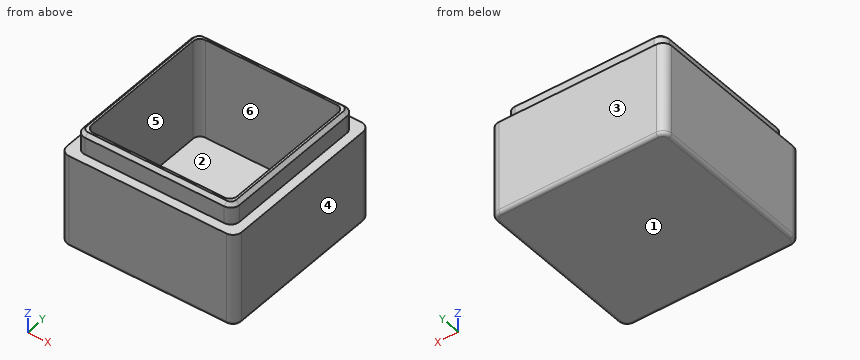
from build123d import *

# Parameters (mm, degrees)
F0_W          = 50.5
F0_H          = 50.5
F1_DEPTH      = 27
F2_W          = 45.2
F2_H          = 45.2
F3_DEPTH      = 6
F4_W          = 42
F4_H          = 42
F5_DEPTH      = 6
F5_DEPTH_BACK = 23
F6_R          = 2.5
F7_R          = 2
F8_SIZE       = 1
F9_R          = 1


with BuildPart() as f1:
    # F0 (on Top) → F1 (new body)
    with BuildSketch(Plane.XY):
        Rectangle(F0_W, F0_H)
    extrude(amount=F1_DEPTH)

    # F2 (on face) → F3 (join)
    with BuildSketch(Plane.XY.offset(27)):
        Rectangle(F2_W, F2_H)
    extrude(amount=F3_DEPTH)

    # F4 (on face) → F5 (cut, two sides)
    with BuildSketch(Plane.XY.offset(27)) as f5_sk:
        Rectangle(F4_W, F4_H)
    extrude(amount=F5_DEPTH, mode=Mode.SUBTRACT)
    extrude(f5_sk.sketch, amount=-F5_DEPTH_BACK, mode=Mode.SUBTRACT)

    # F6
    f6_edges = [f1.edges().sort_by_distance(p)[0] for p in [
        (-25.25, 25.25, 13.5),
        (-25.25, -25.25, 13.5),
        (25.25, -25.25, 13.5),
        (25.25, 25.25, 13.5),
        (-22.6, 22.6, 30),
        (-22.6, -22.6, 30),
        (22.6, -22.6, 30),
        (22.6, 22.6, 30),
    ]]
    fillet(f6_edges, radius=F6_R)

    # F7
    f7_edges = [f1.edges().sort_by_distance(p)[0] for p in [
        (-21, 21, 18.5),
        (21, 21, 18.5),
        (21, -21, 18.5),
        (-21, -21, 18.5),
    ]]
    fillet(f7_edges, radius=F7_R)

    # F8
    f8_edges = [f1.edges().sort_by_distance(p)[0] for p in [
        (-22.6, 0, 33),
    ]]
    chamfer(f8_edges, length=F8_SIZE)

    # F9
    f9_edges = [f1.edges().sort_by_distance(p)[0] for p in [
        (0, 25.25, 0),
    ]]
    fillet(f9_edges, radius=F9_R)


solid = f1.part
Check sheet for the modelled part. Datum: model origin and axes. Units: mm. Face numbers are marked on the shaded views. A direction names the side the tool comes from. Give positions to 0.01 mm unless a question says otherwise; leave off trailing zeros. Write each loop counter-clockwise with the first axis right and the second up, starting at its lowest first coordinate (ties: lowest second). Pieces come first, ordered by that corner, then holes. Notation, with made-up numbers: (24.5, 51.5) -> (69.5, 51.5) arc R10 cw to (69.5, 61.5) -> close; hole circle Ø6 at (87, 64.25). An arc over 180 degrees is marked (long way). Use one line per item in the form item = value. Start each with the question number.
1. Thickness scan on line 1 along X through (y, z) = (-15, 20); line 2 along X through (y, z) = (-2, 30). Record the ranges inside material, lowest first. Write a range as from..to.
2. Access from +Z, -Z, +X, -X, +Y, -Y to the whole of each face (thin tool, end or side, straight path). Record for the marked faces 1 and 2.
3. Section check B-B (y = -3). Record the cut outline in (x, z), and give its area (3 significant figures).
4. Mould release check, pull along X, two halves, no side actions. Record for the marked faces 3, 4, 5 and 6: pulls with the +X half, pulls with the -X half, needs draft (parallel to the pull), parting line crosses it, or undercut.
5. Go/stop test with flat-tipped pins: P1, Ø8, axis at x = -15, y = -7, coming from the +Z side; P2, Ø2.5, axis at y = 6.5, z = 29, coming from the -X side; P3, Ø2.5, axis at x = 9, z = 28.5, coming from the +Y side. Record where each tip stops, or that it passes through.
6. Section check A-A (z = 11). Record the cut outline in (x, y).
Conclusion:
q1.line_1 = -25.25..-21, 21..25.25
q1.line_2 = -22.6..-21, 21..22.6
q2.face_1 = -Z, +X, -X, +Y, -Y
q2.face_2 = +Z
q3.outline = (-25.25, 1) arc R1 ccw to (-24.25, 0) -> (24.25, 0) arc R1 ccw to (25.25, 1) -> (25.25, 27) -> (22.6, 27) -> (22.6, 32) -> (21.6, 33) -> (21, 33) -> (21, 4) -> (-21, 4) -> (-21, 33) -> (-21.6, 33) -> (-22.6, 32) -> (-22.6, 27) -> (-25.25, 27) -> close
q3.area = 415 mm²
q4.face_3 = needs draft
q4.face_4 = pulls with the +X half
q4.face_5 = undercut
q4.face_6 = undercut
q5.P1 = 4
q5.P2 = -22.6
q5.P3 = 22.6
q6.outline = (-25.25, -22.75) arc R2.5 ccw to (-22.75, -25.25) -> (22.75, -25.25) arc R2.5 ccw to (25.25, -22.75) -> (25.25, 22.75) arc R2.5 ccw to (22.75, 25.25) -> (-22.75, 25.25) arc R2.5 ccw to (-25.25, 22.75) -> close; hole (-21, -19) arc R2 ccw to (-19, -21) -> (19, -21) arc R2 ccw to (21, -19) -> (21, 19) arc R2 ccw to (19, 21) -> (-19, 21) arc R2 ccw to (-21, 19) -> close
